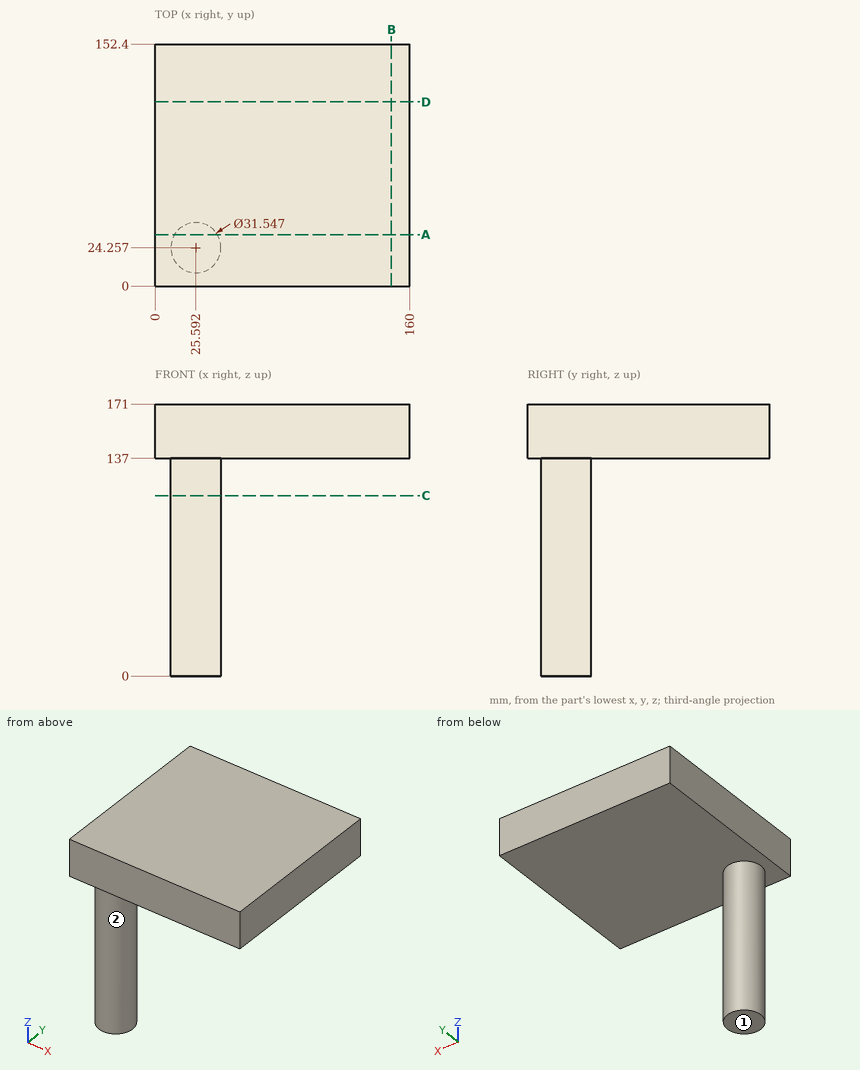
Job drawing, mm, ordinate dimensions from the low corner. One solid piece. A direction names the side the tool comes from. Round coordinates to 2 decimals unless told otherwise and drop trailing zeros. Loops run counter-clockwise (first coordinate to the right, second up) from the corner with the lowest first, then second, coordinate; pieces in that order, holes last. Notation, with made-up numbers: (-33.5, 49) -> (-13.5, 49) arc R31 cw to (-13.5, 85) -> close; hole circle Ø5 at (4.5, 86). An arc over 180 degrees is marked (long way). Use a Markdown table: item, result.
1) Cut at D-D, the plane y = 116. List the corners of the cut face in (x, z).
The answers:
| item | result |
|---|---|
| outline | (0, 137) -> (160, 137) -> (160, 171) -> (0, 171) -> close |
2) Probe line 1 (Z direction, x = 92, y = 20); line 2 (Y direction, x = 24.5, z = 77); line 3 (Y direction, x = 16, z = 50) (1 decimal). List the from-to ranges inside material, lowest first. Write a range as [from, to].
The answers:
| item | result |
|---|---|
| line 1 | z = [137, 171] |
| line 2 | y = [8.52, 39.99] |
| line 3 | y = [11.7, 36.8] |
3) Cut at B-B, the plane x = 148.5. List the corners of the cut face in (y, z), and give its area (3 significant figures).
The answers:
| item | result |
|---|---|
| outline | (0, 137) -> (152.4, 137) -> (152.4, 171) -> (0, 171) -> close |
| area | 5,180 mm2 |
4) Cut at C-C, the plane z = 113.5. List the corners of the cut face in (x, y) (1 decimal).
The answers:
| item | result |
|---|---|
| outline | circle Ø31.5 at (25.6, 24.3) |
5) Drop flat-ended pins along their axis: pin 1 Ø6 at (x, z) = (38, 31.5) entering from +Y; pin 2 Ø8 at (y, z) = (18, 134) entering from +X; pin 3 Ø4 at (x, z) = (37.5, 78) entering from -Y; pin 4 Ø8 at (x, z) = (29, 127.5) entering from +Y. Give the stop position or say it passes through.
The answers:
| item | result |
|---|---|
| pin 1 | stops at y = 36.92 |
| pin 2 | stops at x = 160 |
| pin 3 | stops at y = 11.98 |
| pin 4 | stops at y = 40.03 |
6) Cut at A-A, the plane y = 32.5. List the corners of the cut face in (x, z).
The answers:
| item | result |
|---|---|
| outline | (0, 137) -> (12.14, 137) -> (12.14, 0) -> (39.04, 0) -> (39.04, 137) -> (160, 137) -> (160, 171) -> (0, 171) -> close |
7) Tool access for the marked faces 1 and 2: list every direction of +Z, -Z, +X, -X, +Y, -Y with a clear straight run to the whole face (end or side of a thin tool).
The answers:
| item | result |
|---|---|
| face 1 | -Z, +X, -X, +Y, -Y |
| face 2 | -Z |
